from build123d import *

# Parameters (mm, degrees)
SKETCH_1_W      = 29
SKETCH_1_H      = 29
EXTRUDE_1_DEPTH = 65
SHELL_1_T       = -2


with BuildPart() as part:
    # Эскиз1 → Бобышка-Вытянуть1 (new body)
    with BuildSketch(Plane(origin=(0, 0, 0), x_dir=(1, 0, 0), z_dir=(0, 1, 0))):
        Rectangle(SKETCH_1_W, SKETCH_1_H)
    extrude(amount=EXTRUDE_1_DEPTH)

    # Оболочка1
    shell_1_openings = [part.faces().sort_by_distance(p)[0] for p in [
        (0, 65, 0),
        (0, 0, 0),
    ]]
    offset(amount=SHELL_1_T, openings=shell_1_openings, kind=Kind.INTERSECTION)


solid = part.part
Design review of the part built by this model. Coordinates are the model's own, in mm. A direction names the side the tool comes from. Coordinates: 2 decimals unless noted, no trailing zeros. Order: outer loops, then holes, each group sorted by start corner. A loop starts at its lowest first (then second) coordinate and runs counter-clockwise, first axis right, second up. Notation, with made-up numbers: (16.5, 57.5) -> (32.5, 57.5) arc R28 cw to (32.5, 96.5) -> close; hole circle Ø9 at (-34, 12.5). An arc over 180 degrees is marked (long way). Use one line per item in the form item = value. Start each with the question number.
(1) For faces 1 (the flat face through (-12.5, 32, 0)), 2 (the flat face through (14.5, 32, 0)), list the 3-axis set-ups (+Z, -Z, +X, -X, +Y, -Y) from which the entire face can be reached by the end or side of a thin tool; tool diameter is ignored.
(2) Add section C-C on x = 1. State the section outline as (y, z) points, plus the area to 3 significant figures.
(3) Add section B-B on y = 52. State the section outline as (x, z) points.
(4) Add section A-A on z = -9. State the section outline as (x, y) points.
(5) For probe 1 along Z at (x, y) = (10.5, 25.5), list the stretches that pass through material, from the lowest coordinate up.
(6) Insertion check: pin 1 (3 mm diameter, centred on x = -3.5, z = 9.5, fed in from +Y). The pin has a flat end and moves straight along its axis. Give the tip position at first contact, or say it passes through.
(7) The part is to be moulded in two halves that separate along Z. For faces 3 (the flat face through (0, 32, -14.5)), 4 (the flat face through (0, 32, 12.5)), 5 (the flat face through (-14.5, 32, 0)), say which applies: +Z half, -Z half, draft (parallel to the pull), parting line (faces both ways), or undercut.
Answer block:
q1.face_1 = +Y, -Y
q1.face_2 = +Z, -Z, +X, +Y, -Y
q2.outline = (0, -14.5) -> (65, -14.5) -> (65, -12.5) -> (0, -12.5) -> close; (0, 12.5) -> (65, 12.5) -> (65, 14.5) -> (0, 14.5) -> close
q2.area = 260 mm²
q3.outline = (-14.5, -14.5) -> (14.5, -14.5) -> (14.5, 14.5) -> (-14.5, 14.5) -> close; hole (-12.5, -12.5) -> (12.5, -12.5) -> (12.5, 12.5) -> (-12.5, 12.5) -> close
q4.outline = (-14.5, 0) -> (-12.5, 0) -> (-12.5, 65) -> (-14.5, 65) -> close; (12.5, 0) -> (14.5, 0) -> (14.5, 65) -> (12.5, 65) -> close
q5.probe_1 = -14.5 to -12.5, 12.5 to 14.5
q6.pin_1 = through
q7.face_3 = -Z half
q7.face_4 = undercut
q7.face_5 = draft
